Read the model definition and answer for the solid it produces. Units are mm, in the model's axes. Face numbers are marked on the shaded views. A direction names the side the tool comes from. Give positions to 0.01 mm unless a question says otherwise; leave off trailing zeros. Loops run counter-clockwise (first coordinate to the right, second up) from the corner with the lowest first, then second, coordinate; pieces in that order, holes last. Notation, with made-up numbers: (35.25, -19) - (79.25, -19) arc R27 ccw to (79.25, 10) - close; hole circle Ø5 at (32, -27). An arc over 180 degrees is marked (long way). Put each result on its own line as item: value. Start each with the question number.
1. For the marked faces 1 and 2, determine the directions among +Z, -Z, +X, -X, +Y, -Y from which every point of the face is accessible in a straight line to the end or side of a thin tool.
2. A cutting plane is placed at D-D, the plane x = -355.5. Determine the outline of the cut face in (y, z).
3. A cutting plane is placed at C-C, the plane x = -358.75. Determine the outline of the cut face in (y, z).
4. Given pin 1 Ø1 at (x, z) = (-366.5, -17) entering from +Y; pin 2 Ø5 at (x, z) = (-354, 17) entering from +Y; pin 3 Ø3 at (x, y) = (-353.5, -12.5) entering from -Z, each flat-ended and moving along its own axis, determine where each tip first touches the part or whether it passes through.
5. Consider L1, parallel to Z at x = -356.5, y = -0.5; L2, parallel to Z at x = -368.25, y = 0; L3, parallel to X at y = -21.5, z = -10. Determine where each line is inside the solid, lowest interval first. Write a range as from..to.
6. A cutting plane is placed at B-B, the plane x = -364.75. Determine the outline of the cut face in (y, z).
```python
from build123d import *

# Parameters (mm, degrees)
ZAOBLIT1_R               = 0.5
ODEBRAT_START            = -8
ODEBRAT_VYSUNUT_M2_DEPTH = 8.026334


with BuildPart() as part:
    # Skica1 → Rotovat1 (revolve)
    with BuildSketch(Plane.XY):
        Polygon((-351.05, 24), (-353.05, 24), (-353.05, 22), (-358.05, 22), (-358.05, 24), (-360.55, 24), (-360.55, 27), (-365.55, 27), (-365.55, 20), (-367.05, 20), (-367.55, 21), (-370.55, 21), (-370.55, 19), (-370.55, 17), (-363.55, 17), (-363.55, 19), (-351.05, 19), align=None)
    revolve(axis=Axis((-379.936676629, 0, 0), (1, 0, 0)))

    # Zaoblit1
    zaoblit1_edges = [part.edges().sort_by_distance(p)[0] for p in [
        (-363.55, -19, 0),
    ]]
    fillet(zaoblit1_edges, radius=ZAOBLIT1_R)

    # Skica3 → Odebrat vysunutím2 (cut)
    with BuildSketch(Plane(origin=(0, -19, 0), x_dir=(1, 0, 0), z_dir=(0, 1, 0)).offset(ODEBRAT_START)):
        with BuildLine():
            Line((-353.05, -1), (-361.55, -1))
            ThreePointArc((-361.55, -1), (-362.55, 0), (-361.55, 1))
            Line((-361.55, 1), (-353.05, 1))
            ThreePointArc((-353.05, 1), (-352.05, 0), (-353.05, -1))
        make_face()
    extrude(amount=ODEBRAT_VYSUNUT_M2_DEPTH, mode=Mode.SUBTRACT)


solid = part.part
```
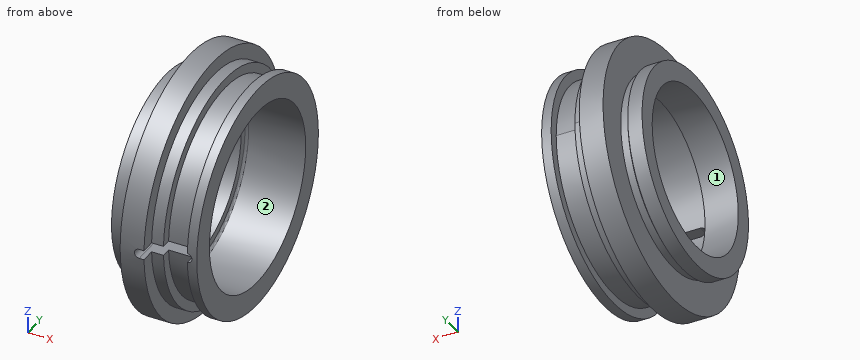
Return value:
1. face 1: +X, -X
1. face 2: +X
2. outline: (-21.98, -1) arc R22 ccw (long way) to (-21.98, 1) - (-18.97, 1) arc R19 cw (long way) to (-18.97, -1) - close
3. outline: (-23.98, -1) arc R24 ccw (long way) to (-23.98, 1) - (-18.97, 1) arc R19 cw (long way) to (-18.97, -1) - close
4. pin 1: stops at y = 11.3
4. pin 2: stops at y = 18.98
4. pin 3: stops at z = -21.29
5. L1: z = -21.99..-18.99, 18.99..21.99
5. L2: z = -21..-17, 17..21
5. L3: x = -365.55..-358.05, -353.05..-351.05
6. outline: circle Ø54 at (0, 0); hole circle Ø34 at (0, 0)
